Design review of the part shown in the three views and the two pictorial views. Dimensions are in mm from the part's minimum x, y and z. A direction names the side the tool comes from. Coordinates: 2 decimals unless noted, no trailing zeros. Write each loop counter-clockwise with the first axis right and the second up, starting at its lowest first coordinate (ties: lowest second). Pieces come first, ordered by that corner, then holes. Notation, with made-up numbers: M -2.75,36 L 34.25,36 A19 ccw 34.25,42 Z; hole C -23.5,65.5 d2. An arc over 180 degrees is marked long. One line per question, with ' | ' between items.
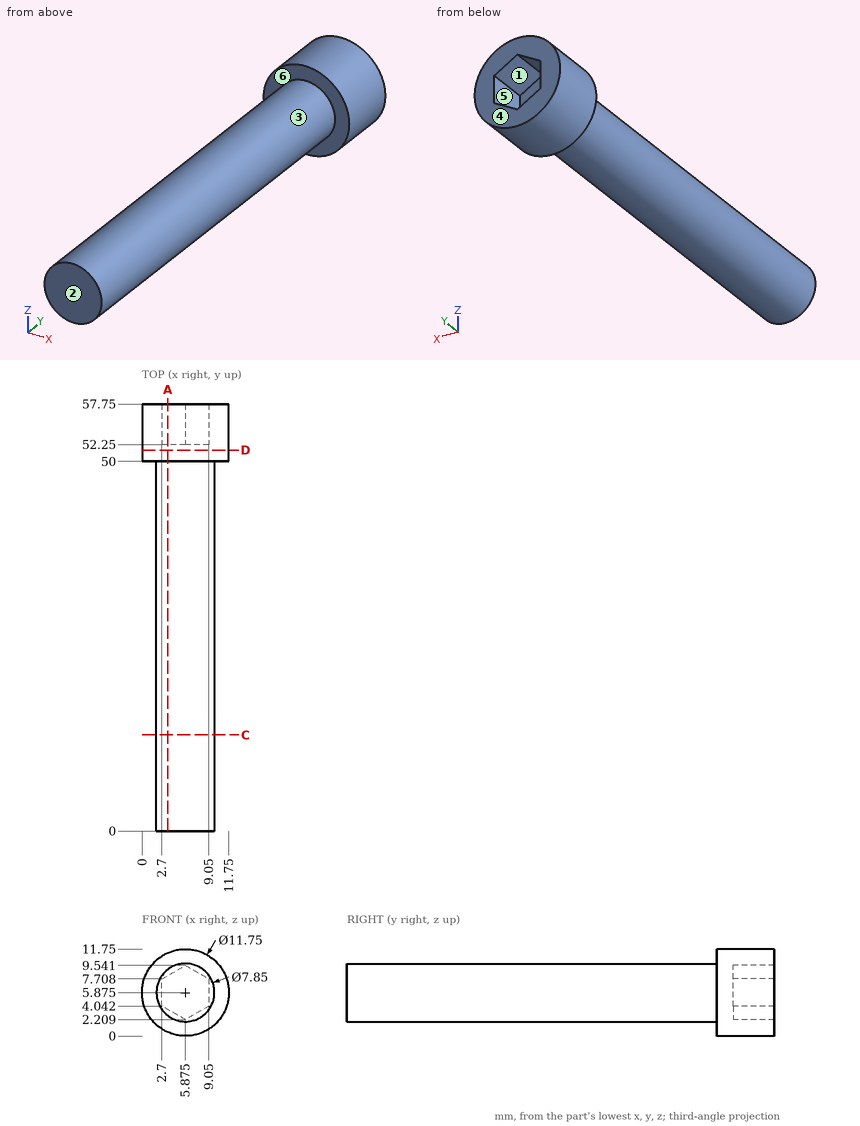
1. Machinability: for the marked faces 4, 5 and 6, which of the approach directions +Z, -Z, +X, -X, +Y, -Y give a long, thin tool a straight path to every point of the face, cutting with its end or side? Answer none if there is none.
Computed values:
face 4: +Z, -Z, +X, -X, +Y | face 5: +Y | face 6: -Y
2. For line 1 along X through (y, z) = (34, 6); line 2 along Y through (x, z) = (7, 9.75); line 3 along Y through (x, z) = (5.75, 8.5), list the stretches that pass through material, from the lowest coordinate up.
Computed values:
line 1: x = 1.95 to 9.8 | line 2: y = 50 to 57.75 | line 3: y = 0 to 52.25
3. Take a section at C-C on y = 13. State the section outline as (x, z) points (3 decimals), plus the area to 3 significant figures.
Computed values:
outline: C 5.875,5.875 d7.85 | area: 48.4 mm2
4. Draft analysis for pull direction Z (two halves, no side actions). For the marked faces 1, 2 and 3, state which applies: pulls with the +Z half, pulls with the -Z half, needs draft (parallel to the pull), parting line crosses it, or undercut.
Computed values:
face 1: undercut | face 2: needs draft | face 3: parting line crosses it
5. Take a section at D-D on y = 51.5. State the section outline as (x, z) points (3 decimals), plus the area to 3 significant figures.
Computed values:
outline: C 5.875,5.875 d11.75 | area: 108 mm2
6. Take a section at A-A on x = 3.5. State the section outline as (y, z) points.
Computed values:
outline: M 0,2.75 L 50,2.75 L 50,0.5 L 57.75,0.5 L 57.75,3.58 L 52.25,3.58 L 52.25,8.17 L 57.75,8.17 L 57.75,11.25 L 50,11.25 L 50,9 L 0,9 Z
7. Clearance check with flat-ended pins moving along their axes: P1, Ø1.8, axis at y = 54.5, z = 6.5, coming from the -X side; P2, Ø4, axis at y = 41.5, z = 7.5, coming from the +X side; P3, Ø1.5, axis at x = 2, y = 49, coming from the +Z side. State where each tip first meets the part, or that it passes through.
Computed values:
P1: stops at x = 0 | P2: stops at x = 9.8 | P3: stops at z = 8.25
